Autodesk Fusion 360 part; units mm, degrees
sketch "top view" plane through (0, 0, 0) normal (0, 0, 1) x (1, 0, 0)
  line L0 (-105, 33) -> (-105, -11) construction
  line L1 (-125, 15) -> (-126.282, 15) construction
  line L2 (-126.282, 15) -> (-126.282, 15.368) construction
  line L3 (-126.282, 15.368) -> (-127.5617, 16.726)
  line L4 (-126.282, 15.368) -> (-124.416, 15.368) construction
  line L5 (-127.5617, 16.726) -> (-127.5786, 16.744)
  line L6 (-126.282, 14.632) -> (-127.5617, 13.274)
  line L7 (-127.5617, 13.274) -> (-127.5786, 13.256)
  line L8 (-125, 15) -> (-123.748, 15) construction
  line L9 (-123.748, 15) -> (-123.748, 17.8501) construction
  line L10 (-123.748, 15) -> (-123.748, 12.1499) construction
  line L11 (-123.748, 15) -> (-123.748, 15.461) construction
  line L12 (-123.748, 15) -> (-123.748, 14.539) construction
  arc A0 (-126.282, 14.632) -> (-123.7484, 14.539) centre (-125, 15) ccw
  arc A1 (-123.7484, 15.461) -> (-126.282, 15.368) centre (-125, 15) ccw
  line L13 (-121.9213, 15.461) -> (-120.224, 15.461)
  line L14 (-121.9213, 14.539) -> (-120.224, 14.539)
  arc A2 (-127.5786, 13.256) -> (-123.134, 12.5083) centre (-125, 15) ccw
  arc A3 (-123.134, 17.4917) -> (-127.5786, 16.744) centre (-125, 15) ccw
  arc A4 (-120.224, 14.539) -> (-120.224, 15.461) centre (-120.224, 15) ccw
  line L15 (-125, 15) -> (-123.134, 15) construction
  line L16 (-123.134, 15) -> (-123.134, 17.4917) construction
  line L17 (-123.134, 17.4917) -> (-120.5917, 17.2693)
  line L18 (-123.134, 17.4917) -> (-120.582, 17.4917) construction
  line L19 (-123.134, 12.5083) -> (-120.5917, 12.7307)
  line L20 (-118.9667, 18.8943) -> (-119.4889, 24.8635)
  line L21 (-118.9667, 18.8943) -> (-111.0132, 18.8943) construction
  line L22 (-123.134, 17.4917) -> (-118.737, 17.4917) construction
  line L23 (-118.9667, 18.8942) -> (-118.9667, 18.8942)
  arc A5 (-120.5917, 17.2693) -> (-118.9667, 18.8943) centre (-120.461, 18.7636) ccw
  line L24 (-119.4004, 17.7029) -> (-121.3897, 15.7137) construction
  line L25 (-119.4004, 17.7029) -> (-116.4958, 14.7981) construction
  line L26 (-123.748, 15.461) -> (-121.9213, 15.461)
  line L27 (-123.748, 14.539) -> (-121.9213, 14.539)
  arc A6 (-117.4582, 21.9535) -> (-116.9972, 21.4925) centre (-116.9972, 21.9535) ccw
  line L28 (-116.9972, 20.106) -> (-116.9972, 11.6268) construction
  arc A7 (-115.0277, 18.8943) -> (-113.4026, 17.2693) centre (-113.5334, 18.7636) ccw
  line L29 (-113.4026, 17.2693) -> (-105, 17.2693)
  line L30 (-105, 33) -> (-105, -11) construction
  line L31 (-96.5974, 17.2693) -> (-105, 17.2693)
  arc A8 (-96.5974, 17.2693) -> (-94.9723, 18.8943) centre (-96.4667, 18.7636) ccw
  line L32 (-94.9723, 18.8943) -> (-95.2773, 22.3803)
  line L33 (-93.0028, 20.106) -> (-93.0028, 11.6268) construction
  line L34 (-91.7911, 18.8943) -> (-98.9868, 18.8943) construction
  line L35 (-91.0333, 17.2692) -> (-93.5042, 14.7981) construction
  line L36 (-91.0333, 17.4917) -> (-91.263, 17.4917) construction
  line L37 (-82.4383, 16.726) -> (-82.4214, 16.744)
  line L38 (-83.718, 15) -> (-83.718, 15.368) construction
  arc A9 (-86.866, 12.5083) -> (-86.252, 12.1499) centre (-85, 15) ccw
  line L39 (-91.0333, 18.8943) -> (-91.0333, 18.8943)
  line L40 (-82.4383, 13.274) -> (-82.4214, 13.256)
  spline S0 degree 5 poles (-120.5917, 12.7307) (-119.326, 12.8736) (-116.8026, 13.1337) (-113.042, 13.4467) (-108.0773, 13.7071) (-101.9596, 13.7532) (-97.0107, 13.5402) (-93.3168, 13.2188) (-90.8349, 12.9243) (-89.5363, 12.7482) (-89.4083, 12.7307) knots 0 0 0 0 0 0 0.1 0.2 0.3 0.4 0.5 0.51094 0.51094 0.51094 0.51094 0.51094 0.51094
  line L41 (-92.4447, 13.1474) -> (-86.3719, 12.3139)
  line L42 (-123.748, 14.539) -> (-123.7484, 14.539)
  line L43 (-123.748, 15.461) -> (-123.7484, 15.461)
  line L44 (-116.5362, 25.4775) -> (-116.5362, 25.4779)
  line L45 (-117.4582, 25.4775) -> (-117.4582, 25.4779)
  line L46 (-115.0277, 18.8943) -> (-115.0278, 18.8929)
  line L47 (-118.9704, 18.9365) -> (-118.9667, 18.8943)
  line L48 (-119.4004, 17.7029) -> (-116.9972, 20.106) construction
  line L49 (-125, 15) -> (-93.0028, 15) construction
  line L50 (-93.0028, 15) -> (-125, 15) construction
  line L51 (-91.7911, 18.8943) -> (-93.0028, 20.106) construction
  arc A10 (-114.5054, 24.8635) -> (-115.2532, 29.3081) centre (-116.9972, 26.7295) ccw
  arc A11 (-118.7411, 29.3081) -> (-119.4889, 24.8635) centre (-116.9972, 26.7295) ccw
  arc A12 (-117.3652, 28.0115) -> (-117.4582, 25.4779) centre (-116.9972, 26.7295) ccw
  arc A13 (-116.5362, 25.4779) -> (-116.6292, 28.0115) centre (-116.9972, 26.7295) ccw
  line L52 (-116.5362, 23.6508) -> (-116.5362, 21.9535)
  arc A14 (-117.4582, 21.9535) -> (-116.5362, 21.9535) centre (-116.9972, 21.9535) ccw
  line L53 (-117.4582, 23.6508) -> (-117.4582, 21.9535)
  line L54 (-116.5362, 25.4779) -> (-116.5362, 23.6508)
  line L55 (-117.4582, 25.4779) -> (-117.4582, 23.6508)
  line L56 (-115.2532, 29.3081) -> (-116.6292, 28.0115)
  line L57 (-117.3652, 28.0115) -> (-118.7411, 29.3081)
  line L58 (-114.5054, 24.8635) -> (-115.0278, 18.8929)
  arc A15 (-90.5111, 24.8635) -> (-91.2589, 29.3081) centre (-93.0028, 26.7295) ccw
  arc A16 (-94.7468, 29.3081) -> (-95.4946, 24.8635) centre (-93.0028, 26.7295) ccw
  line L59 (-94.7468, 29.3081) -> (-93.3708, 28.0115)
  line L60 (-92.6348, 28.0115) -> (-91.2589, 29.3081)
  arc A17 (-92.5418, 25.4779) -> (-92.6348, 28.0115) centre (-93.0028, 26.7295) ccw
  arc A18 (-93.3708, 28.0115) -> (-93.4638, 25.4779) centre (-93.0028, 26.7295) ccw
  line L61 (-93.4638, 25.4779) -> (-93.4638, 23.6508)
  line L62 (-92.5418, 25.4779) -> (-92.5418, 23.6508)
  line L63 (-91.0333, 18.8943) -> (-90.5111, 24.8635)
  line L64 (-92.5418, 23.6508) -> (-92.5418, 21.9535)
  line L65 (-93.4638, 23.6508) -> (-93.4638, 21.9535)
  arc A19 (-93.4638, 21.9535) -> (-92.5418, 21.9535) centre (-93.0028, 21.9535) ccw
  arc A20 (-91.0333, 18.8943) -> (-89.4083, 17.2693) centre (-89.539, 18.7636) ccw
  line L66 (-86.866, 17.4917) -> (-89.4083, 17.2693)
  arc A21 (-82.4214, 16.744) -> (-86.866, 17.4917) centre (-85, 15) ccw
  arc A22 (-83.718, 15.368) -> (-86.2516, 15.461) centre (-85, 15) ccw
  arc A23 (-86.2516, 14.539) -> (-83.718, 14.632) centre (-85, 15) ccw
  arc A24 (-86.866, 12.5083) -> (-82.4214, 13.256) centre (-85, 15) ccw
  line L67 (-88.0787, 14.539) -> (-89.776, 14.539)
  line L68 (-88.0787, 15.461) -> (-89.776, 15.461)
  arc A25 (-89.776, 15.461) -> (-89.776, 14.539) centre (-89.776, 15) ccw
  line L69 (-95.4946, 24.8635) -> (-94.9722, 18.8929)
  line L70 (-86.866, 12.5083) -> (-89.4083, 12.7307)
  line L71 (-88.0787, 15.461) -> (-86.2516, 15.461)
  line L72 (-88.0787, 14.539) -> (-86.2516, 14.539)
  line L73 (-83.718, 15.368) -> (-82.4214, 16.744)
  line L74 (-83.718, 14.632) -> (-82.4214, 13.256)
  point P0 (-95.4946, 24.8635)
  point P1 (-94.7468, 29.3081)
  point P2 (-93.0028, 26.7295)
  point P3 (-88.6103, 15.7137)
  dimension "d3" = 6.226
  dimension "d4" = 1.282
  dimension "d5" = 0.368
  dimension "d6" = 133.3
  dimension "d7" = 1.866
  dimension "d8" = 1.252
  dimension "d9" = 0.461
  dimension "d10" = 0.461
  dimension "d11" = 3.524
  dimension "d12" = 0.922
  dimension "d13" = 1.866
  dimension "d14" = 2.552
  dimension "d15" = 5
  dimension "d16" = 3
  dimension "d17" = 95
  dimension "d18" = 5.992
  dimension "d20" = 4.397
  dimension "d24" = 0.922
  dimension "d25" = 6.226
  dimension "d28" = 0.922
extrude "Extrude1" add sketch "top view" along normal blind 1.5 contours L3 L5 L6 L7 A0 A1 L13 L14 A2 A3 A4 L17 L19 L20 A5 L26 L27 A6 A7 L29 L31 A8 L32 L37 A9 L40 S0 L47 A10 A11 A12 A13 L52 A14 L53 L54 L55 L56 L57 L58 A15 A16 L59 L60 A17 A18 L61 L62 L63 L64 L65 A19 A20 L66 A21 A22 A23 A24 L67 L68 A25 L69 L70 L71 L72 L73 L74 makes body 1
copy_body "Body->Comp1" bodies 1 removing the originals makes body 2 in component "Piesa_5 (1)"
component "Piesa_5 (1)" placed x (1, 0, 0) y (0, 1, 0) z (0, 0, 1) at (0, 0, 0)
equation "d3 = 3.113 mm + 3.113 mm"
equation "d12 = 0.461 mm + 0.461 mm"
equation "d24 = 0.461 mm + 0.461 mm"
equation "d25 = 3.113 mm + 3.113 mm"
equation "d28 = 0.461 mm + 0.461 mm"
Could you check a few things on this model? Use its own coordinates, in mm. A direction names the side the tool comes from. Give positions to 0.01 mm unless a question says otherwise; leave off trailing zeros. Order: outer loops, then holes, each group sorted by start corner. A loop starts at its lowest first (then second) coordinate and runs counter-clockwise, first axis right, second up.
1. I need wall thicknesses on L1, parallel to X at y = 18.75, z = 0.1; L2, parallel to X at y = 23.25, z = 0.75; L3, parallel to X at y = 22.75, z = 0.55. Which ranges of each line are inside material? Lowest first, please.
Answers below:
L1: x = -118.96 to -115.03, -94.97 to -91.04
L2: x = -119.35 to -117.46, -116.54 to -114.65, -95.35 to -93.46, -92.54 to -90.65
L3: x = -119.3 to -117.46, -116.54 to -114.69, -95.31 to -93.46, -92.54 to -90.7
2. Suppose I cut it at C-C (y = 24). Write out the boundary of the cut face in (x, z).
Answers below:
outline: (-119.41, 0) - (-117.46, 0) - (-117.46, 1.5) - (-119.41, 1.5) - close; (-116.54, 0) - (-114.58, 0) - (-114.58, 1.5) - (-116.54, 1.5) - close; (-95.42, 0) - (-93.46, 0) - (-93.46, 1.5) - (-95.42, 1.5) - close; (-92.54, 0) - (-90.59, 0) - (-90.59, 1.5) - (-92.54, 1.5) - close
3. Suppose I cut it at B-B (y = 27.5). Write out the boundary of the cut face in (x, z).
Answers below:
outline: (-120.01, 0) - (-118.09, 0) - (-118.09, 1.5) - (-120.01, 1.5) - close; (-115.91, 0) - (-113.98, 0) - (-113.98, 1.5) - (-115.91, 1.5) - close; (-96.02, 0) - (-94.09, 0) - (-94.09, 1.5) - (-96.02, 1.5) - close; (-91.91, 0) - (-89.99, 0) - (-89.99, 1.5) - (-91.91, 1.5) - close
4. Thinking about a two-plate mould opening in X: for faces 4 (the flat face through (-126.913, 16.037, 0.74)), 5 (the flat face through (-83.087, 16.038, 0.74)), 6 (the flat face through (-88, 14.539, 1)), 7 (the flat face through (-105, 17, 1.5)), which applies, +X half, -X half, draft (parallel to the pull), parting line (faces both ways), or undercut?
Answers below:
face 4: -X half
face 5: +X half
face 6: undercut
face 7: draft
5. For pin 1 (0.8 mm diameter, centred on x = -87.5, z = 0.5, fed in from +Y); pin 2 (3 mm diameter, centred on x = -115.5, y = 17.5, fed in from -Z); pin 3 (0.8 mm diameter, centred on y = 24.5, z = 1, fed in from +X); pin 4 (0.8 mm diameter, centred on x = -88.5, z = 1, fed in from -Y), each with a flat end and sliding along its axis, tell me the tip position at first contact or that it passes through.
Answers below:
pin 1: stops at y = 17.47
pin 2: stops at z = 0
pin 3: stops at x = -90.48
pin 4: stops at y = 12.62
6. Suppose I cut it at A-A (x = -121.5). Write out the boundary of the cut face in (y, z), plus the area to 3 significant figures.
Answers below:
outline: (12.65, 0) - (14.54, 0) - (14.54, 1.5) - (12.65, 1.5) - close; (15.46, 0) - (17.35, 0) - (17.35, 1.5) - (15.46, 1.5) - close
area: 5.66 mm2
7. Which directions (+Z, -Z, +X, -X, +Y, -Y) give clear straight access to the entire face, cutting with the end or side of a thin tool? Please do faces 1 (the cylindrical face through (-92.993, 21.493, 0.74)), 2 (the flat face through (-88.12, 17.38, 0.74)), 3 (the cylindrical face through (-84.107, 12.018, 0.74)).
Answers below:
face 1: +Z, -Z
face 2: +Z, -Z, +Y
face 3: +Z, -Z, -Y
